The model under review builds one solid part; all positions refer to its coordinate system, in mm. Face numbers are marked on the shaded views. Round coordinates to 2 decimals unless told otherwise and drop trailing zeros.
from build123d import *

# Parameters (mm, degrees)
EXTRUDE_1_DEPTH     = 2
SKETCH_2_R          = 2
CUT_EXTRUDE_1_DEPTH = 3.0000001


with BuildPart() as part:
    # Эскиз1 → Бобышка-Вытянуть1 (new body)
    with BuildSketch(Plane.XY):
        with BuildLine():
            Line((0, 0), (40, 0))
            add(Edge.make_bspline(
                [(40, 0), (-21.389317784, -56.818064534), (-6.67027027, -150)],
                knots=[0, 0, 0, 1, 1, 1], degree=2))
            Line((-6.67027027, -150), (-11.67027027, -150))
            add(Edge.make_bspline(
                [(0, 0), (-49.854113681, -63.235965622), (-11.67027027, -150)],
                knots=[0, 0, 0, 1, 1, 1], degree=2))
        make_face()
    extrude(amount=EXTRUDE_1_DEPTH)

    # Эскиз2 → Вырез-Вытянуть1 (cut, through all)
    with BuildSketch(Plane.XY.offset(2)):
        with Locations((5, -5)):
            Circle(SKETCH_2_R)
        with Locations((25, -5)):
            Circle(SKETCH_2_R)
        with Locations((-9.67027027, -147.5)):
            Circle(SKETCH_2_R)
    extrude(amount=-CUT_EXTRUDE_1_DEPTH, mode=Mode.SUBTRACT)


solid = part.part
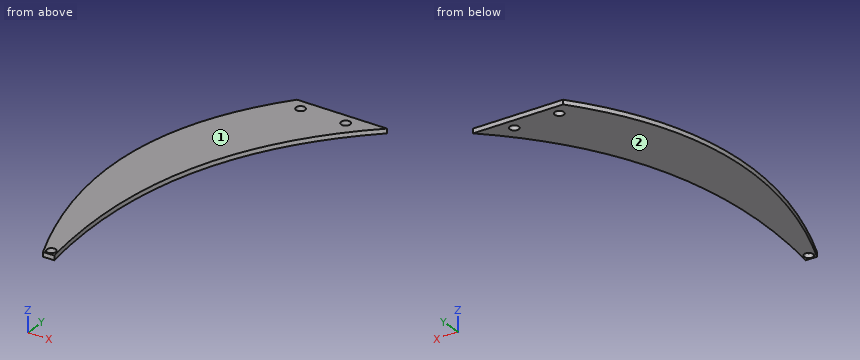
(1) Clearance check with flat-ended pins moving along their axes: P1, Ø2.5, axis at x = -9.67, y = -147.5, coming from the +Z side; P2, Ø1, axis at x = -19, z = 1, coming from the +Y side. State where each tip first meets the part, or that it passes through.
(2) The part is to be moulded in two halves that separate along Z. For the marked faces 1 and 2, say which applies: pulls with the +Z half, pulls with the -Z half, needs draft (parallel to the pull), parting line crosses it, or undercut.
(3) We need section A-A (z = 0.55). Count the separate pieces of the cut face and the enclosed holes in it, and give its area (3 significant figures).
(4) To check wall thickness, follow L1, parallel to Y at x = 5, z = 0.5; L2, parallel to Y at x = 25.5, z = 1.05; L3, parallel to X at y = -91.5, z = 1.55. State the ranges of each line that lie inside material, in increasing order.
Verdict:
1. P1: passes through
1. P2: stops at y = -30.86
2. face 1: pulls with the +Z half
2. face 2: pulls with the -Z half
3. separate pieces: 1
3. enclosed holes: 3
3. area: 3,400 mm2
4. L1: y = -47 to -7, -3 to 0
4. L2: y = -15.18 to -6.94, -3.06 to 0
4. L3: x = -27.67 to -7.97
